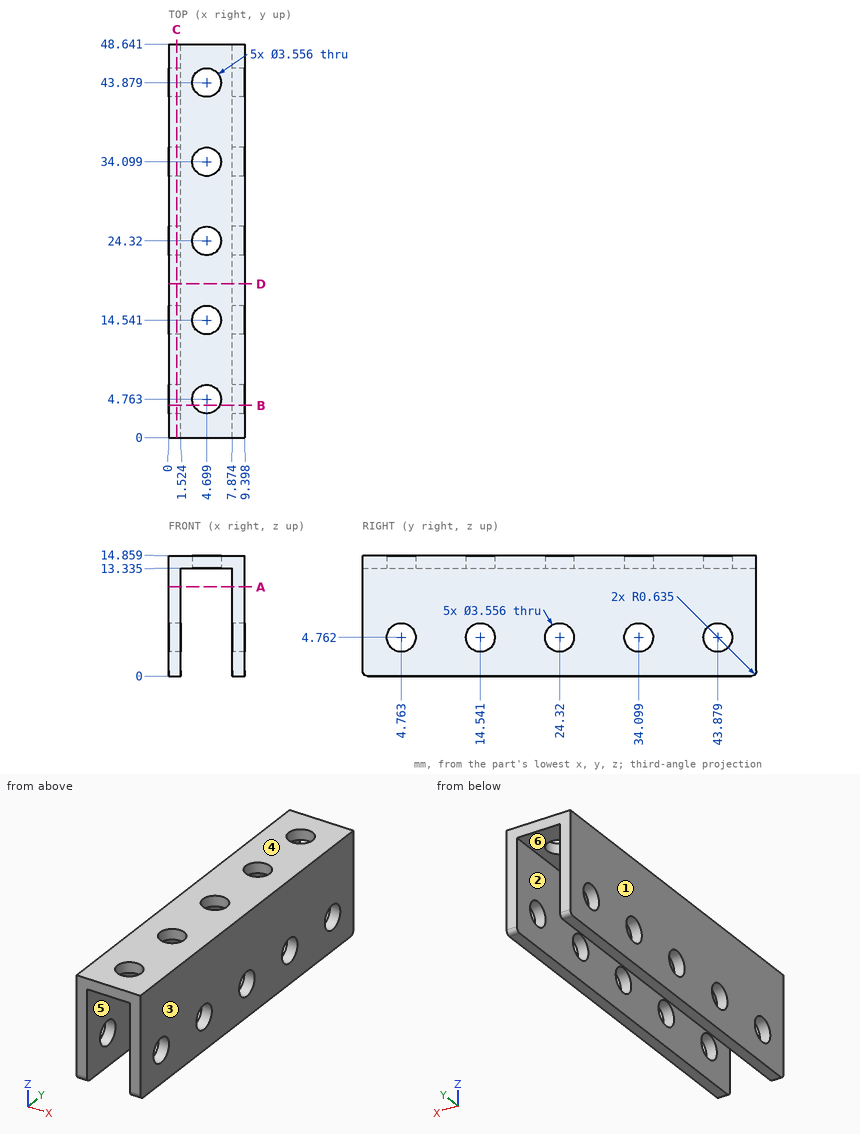
Source: three-view drawing plus pictorial views. Frame: mm from the lowest corner of the part. A direction names the side the tool comes from. Give positions to 0.01 mm unless a question says otherwise; leave off trailing zeros. Loops run counter-clockwise (first coordinate to the right, second up) from the corner with the lowest first, then second, coordinate; pieces in that order, holes last. Notation, with made-up numbers: M 55,-32 L 96,-32 A13 ccw 96,-22 Z; hole C 42.5,23.5 d9. An arc over 180 degrees is marked long. Put each result on its own line as item: value.
Q1. Mould query, pull axis X, two halves, no side actions, for the marked faces 3, 4, 5 and 6. Classes: released by +X, released by -X, zero draft, split by the parting line, or undercut.
Response values:
face 3: released by +X
face 4: zero draft
face 5: undercut
face 6: undercut
Q2. Section D-D (y = 19). Return the cut outline in (x, z) (1 decimal).
Response values:
outline: M 0,0 L 1.5,0 L 1.5,13.3 L 7.9,13.3 L 7.9,0 L 9.4,0 L 9.4,14.9 L 0,14.9 Z
Q3. Pin query (flat end, axial travel): P1, Ø5, axis at x = 5, y = 36, coming from the -Z side (1 decimal); P2, Ø4, axis at y = 43.88, z = 4.76, coming from the -X side; P3, Ø3, axis at x = 6, z = 3, coming from the -Y side. Return the tip coordinate at first contact, or that it passes through.
Response values:
P1: stops at z = 13.3
P2: stops at x = 0
P3: passes through
Q4. Section B-B (y = 4). Return the cut outline in (x, z) (1 decimal).
Response values:
outline: M 0,0 L 1.5,0 L 1.5,3.2 L 0,3.2 Z; M 0,6.4 L 1.5,6.4 L 1.5,13.3 L 3.1,13.3 L 3.1,14.9 L 0,14.9 Z; M 6.3,13.3 L 7.9,13.3 L 7.9,6.4 L 9.4,6.4 L 9.4,14.9 L 6.3,14.9 Z; M 7.9,0 L 9.4,0 L 9.4,3.2 L 7.9,3.2 Z
Q5. Line query: probe 1 along X at (y, z) = (12, 8) (1 decimal); probe 2 along Y at (x, z) = (9.25, 3.75) (1 decimal); probe 3 along Z at (x, y) = (0.75, 43.5) (1 decimal). Output: solid intervals per line, ascending. Write a range as [from, to].
Response values:
probe 1: x = [0, 1.5], [7.9, 9.4]
probe 2: y = [0, 3.3], [6.2, 13.1], [16, 22.9], [25.8, 32.6], [35.6, 42.4], [45.3, 48.6]
probe 3: z = [0, 3], [6.5, 14.9]
Q6. Reachability of the marked faces 1 and 2 from +Z, -Z, +X, -X, +Y, -Y: full face, straight path, thin tool, end or side. Return the list, or none.
Response values:
face 1: +Z, -Z, -X, +Y, -Y
face 2: -Z, +Y, -Y
Q7. Section A-A (z = 11). Return the cut outline in (x, y) (1 decimal).
Response values:
outline: M 0,0 L 1.5,0 L 1.5,48.6 L 0,48.6 Z; M 7.9,0 L 9.4,0 L 9.4,48.6 L 7.9,48.6 Z
Q8. Section C-C (x = 1). Return the cut outline in (y, z) (1 decimal), and give its area (3 significant figures).
Response values:
outline: M 0,0.6 A0.6 ccw 0.6,0 L 48,0 A0.6 ccw 48.6,0.6 L 48.6,14.9 L 0,14.9 Z; hole C 4.8,4.8 d3.6; hole C 14.5,4.8 d3.6; hole C 24.3,4.8 d3.6; hole C 34.1,4.8 d3.6; hole C 43.9,4.8 d3.6
area: 673 mm²
